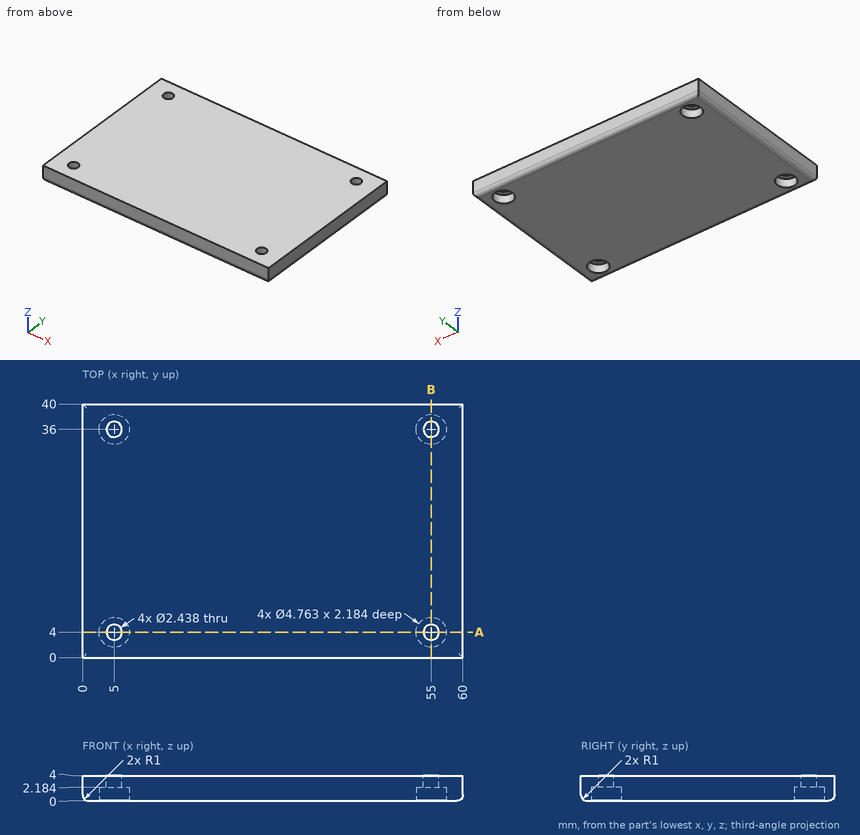
Here's the drawing with two shaded views (mm, measured from the low corner). I have some questions. Give positions to 0.01 mm unless a question says otherwise; leave off trailing zeros. Loops run counter-clockwise (first coordinate to the right, second up) from the corner with the lowest first, then second, coordinate; pieces in that order, holes last. Notation, with made-up numbers: (31.5, 5.5) - (59.5, 5.5) arc R30 ccw to (59.5, 39.5) - close; hole circle Ø1 at (77.25, 73.5). An arc over 180 degrees is marked (long way). Return JSON: item names as keys, results as strings.
1. If I drill on line 1 (Y direction, x = 5, z = 3.3); line 2 (Y direction, x = 5, z = 1.5); line 3 (X direction, y = 5, z = 2.6) (1 decimal), over which ranges is the centre line in solid material (lowest first)?
Output values:
{"line 1": "y = 0 to 2.78, 5.22 to 34.78, 37.22 to 40", "line 2": "y = 0 to 1.62, 6.38 to 33.62, 38.38 to 40", "line 3": "x = 0 to 4.3, 5.7 to 54.3, 55.7 to 60"}
2. I want a section at B-B on x = 55. Please give me the cut outline in (y, z) (1 decimal), and give its area (3 significant figures).
Output values:
{"outline": "(0, 1) arc R1 ccw to (1, 0) - (1.6, 0) - (1.6, 2.2) - (2.8, 2.2) - (2.8, 4) - (0, 4) - close; (5.2, 2.2) - (6.4, 2.2) - (6.4, 0) - (33.6, 0) - (33.6, 2.2) - (34.8, 2.2) - (34.8, 4) - (5.2, 4) - close; (37.2, 2.2) - (38.4, 2.2) - (38.4, 0) - (39, 0) arc R1 ccw to (40, 1) - (40, 4) - (37.2, 4) - close", "area": "130 mm²"}
3. I want a section at A-A on y = 4. Please give me the cut outline in (x, z) (1 decimal), and give its area (3 significant figures).
Output values:
{"outline": "(0, 1) arc R1 ccw to (1, 0) - (2.6, 0) - (2.6, 2.2) - (3.8, 2.2) - (3.8, 4) - (0, 4) - close; (6.2, 2.2) - (7.4, 2.2) - (7.4, 0) - (52.6, 0) - (52.6, 2.2) - (53.8, 2.2) - (53.8, 4) - (6.2, 4) - close; (56.2, 2.2) - (57.4, 2.2) - (57.4, 0) - (59, 0) arc R1 ccw to (60, 1) - (60, 4) - (56.2, 4) - close", "area": "210 mm²"}
4. I'm going to push a flat-ended pin straight in: pin 1 Ø1.4 at (x, y) = (56, 4.5) entering from -Z. Where does the tip first touch, or does it pass through?
Output values:
{"pin 1": "stops at z = 2.18"}
